Autodesk Inventor part; units mm, degrees
ref_plane "YZ Plane" through (0, 0, 0) normal (1, 0, 0) x (0, 1, 0)
ref_plane "XZ Plane" through (0, 0, 0) normal (0, 1, 0) x (-1, 0, 0)
ref_plane "XY Plane" through (0, 0, 0) normal (0, 0, 1) x (1, 0, 0)
sketch "Эскиз1" plane through (0, 0, 0) normal (0, 1, 0) x (-1, 0, 0)
  line L0 (-60, -230) -> (60, -230)
  line L1 (60, -230) -> (60, 230)
  line L2 (60, 230) -> (-60, 230)
  line L3 (-60, 230) -> (-60, -230)
  line L4 (-60, -230) -> (60, 230) construction
  line L5 (60, -230) -> (-60, 230) construction
  point P0 (0, 0)
  dimension "d0" = 120
  dimension "d1" = 460
extrude "Выдавливание1" add sketch "Эскиз1" along normal blind 2
sketch "Эскиз3" plane through (0, 2, 0) normal (0, 1, 0) x (1, 0, 0)
  line L0 (59, -229) -> (-59, -229)
  line L1 (-59, -229) -> (-59, 229)
  line L2 (-59, 229) -> (59, 229)
  line L3 (59, 229) -> (59, -229)
  line L4 (59, -229) -> (-59, 229) construction
  line L5 (-59, -229) -> (59, 229) construction
  line L6 (59, -229) -> (-59, -229)
  line L7 (-59, -229) -> (-59, -116.5)
  line L8 (-59, -116.5) -> (59, -116.5)
  line L9 (59, -116.5) -> (59, -229)
  line L10 (-59, -116.5) -> (59, -116.5)
  line L11 (59, -116.5) -> (59, -114.5)
  line L12 (59, -114.5) -> (-59, -114.5)
  line L13 (-59, -114.5) -> (-59, -116.5)
  line L14 (59, -114.5) -> (-59, -114.5)
  line L15 (-59, -114.5) -> (-59, -2)
  line L16 (-59, -2) -> (59, -2)
  line L17 (59, -2) -> (59, -114.5)
  line L18 (59, -2) -> (-59, -2)
  line L19 (-59, -2) -> (-59, 0)
  line L20 (-59, 0) -> (59, 0)
  line L21 (59, 0) -> (59, -2)
  line L22 (-59, 0) -> (59, 0)
  line L23 (59, 0) -> (59, 112.5)
  line L24 (59, 112.5) -> (-59, 112.5)
  line L25 (-59, 112.5) -> (-59, 0)
  line L26 (-59, 112.5) -> (59, 112.5)
  line L27 (59, 112.5) -> (59, 114.5)
  line L28 (59, 114.5) -> (-59, 114.5)
  line L29 (-59, 114.5) -> (-59, 112.5)
  line L30 (-59, 114.5) -> (59, 114.5)
  line L31 (59, 114.5) -> (59, 229)
  line L32 (59, 229) -> (-59, 229)
  line L33 (-59, 229) -> (-59, 114.5)
  line L34 (-60, 230) -> (-60, -230)
  line L35 (60, -230) -> (60, 230)
  line L36 (-60, -230) -> (60, -230)
  line L37 (60, -230) -> (60, 230)
  line L38 (60, 230) -> (-60, 230)
  line L39 (-60, 230) -> (-60, -230)
  point P0 (0, 0)
  point P1 (59, -116.5)
  point P2 (59, 0)
  point P3 (-59, 112.5)
  dimension "d14" = 118
  dimension "d15" = 458
  dimension "d16" = 112.5
  dimension "d17" = 118
  dimension "d18" = 2
  dimension "d19" = 118
  dimension "d20" = 112.5
  dimension "d21" = 118
  dimension "d22" = 112.5
  dimension "d23" = 118
  dimension "d24" = 2
extrude "Выдавливание3" add sketch "Эскиз3" along normal blind 58 contours L8 L1 L12 L3 | L16 L1 L20 L3 | L24 L1 L28 L3 | L38 L35 L36 L34
properties part number "коробка ардуинкародина"
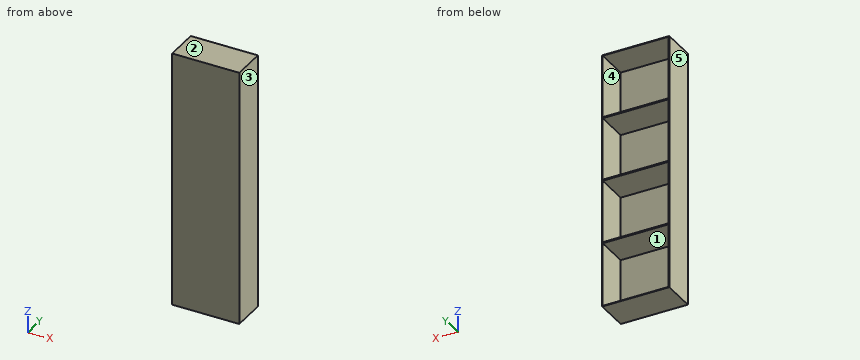
Could you check a few things on this model? Use its own coordinates, in mm. Face numbers are marked on the shaded views. A direction names the side the tool comes from. Give positions to 0.01 mm unless a question says otherwise; leave off trailing zeros. Order: outer loops, then holes, each group sorted by start corner. A loop starts at its lowest first (then second) coordinate and runs counter-clockwise, first axis right, second up.
1. Thinking about a two-plate mould opening in X: for the marked faces 1, 2 and 3, which applies, +X half, -X half, draft (parallel to the pull), parting line (faces both ways), or undercut?
Answers below:
face 1: undercut
face 2: draft
face 3: +X half
2. I need wall thicknesses on L1, parallel to Z at x = -36, y = 27; L2, parallel to X at y = 52.5, z = -80.5; L3, parallel to Y at x = 49, z = -4. Which ranges of each line are inside material? Lowest first, please.
Answers below:
L1: z = -230 to -229, -114.5 to -112.5, 0 to 2, 114.5 to 116.5, 229 to 230
L2: x = -60 to -59, 59 to 60
L3: y = 0 to 2
3. Which directions (+Z, -Z, +X, -X, +Y, -Y) give clear straight access to the entire face, cutting with the end or side of a thin tool? Please do the marked faces 4 and 5.
Answers below:
face 4: +Y
face 5: +Z, -Z, -X, +Y, -Y
4. Suppose I cut it at C-C (x = 10). Write out the boundary of the cut face in (y, z), plus the area to 3 significant figures.
Answers below:
outline: (0, -230) - (60, -230) - (60, -229) - (2, -229) - (2, -114.5) - (60, -114.5) - (60, -112.5) - (2, -112.5) - (2, 0) - (60, 0) - (60, 2) - (2, 2) - (2, 114.5) - (60, 114.5) - (60, 116.5) - (2, 116.5) - (2, 229) - (60, 229) - (60, 230) - (0, 230) - close
area: 1,380 mm2
5. For pin 1 (4 mm diameter, centred on x = -17, z = -150, fed in from +Y), with a flat end and sliding along its axis, tell me the tip position at first contact or that it passes through.
Answers below:
pin 1: stops at y = 2
6. Suppose I cut it at B-B (z = -181.5). Write out the boundary of the cut face in (x, y), plus the area to 3 significant figures.
Answers below:
outline: (-60, 0) - (60, 0) - (60, 60) - (59, 60) - (59, 2) - (-59, 2) - (-59, 60) - (-60, 60) - close
area: 356 mm2
7. Suppose I cut it at A-A (y = 53.5). Write out the boundary of the cut face in (x, z).
Answers below:
outline: (-60, -230) - (60, -230) - (60, 230) - (-60, 230) - close; hole (-59, -229) - (59, -229) - (59, -114.5) - (-59, -114.5) - close; hole (-59, -112.5) - (59, -112.5) - (59, 0) - (-59, 0) - close; hole (-59, 2) - (59, 2) - (59, 114.5) - (-59, 114.5) - close; hole (-59, 116.5) - (59, 116.5) - (59, 229) - (-59, 229) - close
